Verification items for the finished model (mm, model axes). Face numbers are marked on the shaded views. A direction names the side the tool comes from. Coordinates: 2 decimals unless noted, no trailing zeros. Order: outer loops, then holes, each group sorted by start corner. A loop starts at its lowest first (then second) coordinate and runs counter-clockwise, first axis right, second up. Notation, with made-up numbers: (47, 40.25) -> (68, 40.25) arc R7 ccw to (68, 46.25) -> close; hole circle Ø11 at (81.5, 80). An arc over 180 degrees is marked (long way). Write each question's results on one line, items separated by ' | '. Start each with the question number.
(1) Cross-section at A-A on x = -0.5. Enter the section's corners in (y, z).
(2) Set-up check for the marked faces 1, 2 and 3: record each of +Z, -Z, +X, -X, +Y, -Y from which the full face is reachable in a straight line by a thin tool's end or side.
(3) Go/stop test with flat-tipped pins: pin 1 (6 mm diameter, centred on x = 32.5, y = 20, fed in from +Z); pin 2 (0.8 mm diameter, centred on y = 5.5, z = 40.5, fed in from +X); pin 3 (3 mm diameter, centred on y = 33.5, z = -12.5, fed in from -X). Record where each tip stops, or that it passes through.
(4) Cross-section at D-D on x = -16. Enter the section's corners in (y, z).
(5) Cross-section at C-C on y = 31. Enter the section's corners in (x, z), and give its area (3 significant figures).
(6) Thickness scan on probe 1 along X at (y, z) = (30.5, -0.5); probe 2 along Y at (x, z) = (18, 3.5). Record the ranges inside material, lowest first. Write a range as [from, to].
(7) Cross-section at B-B on z = 2. Enter the section's corners in (x, y).
(8) Draft check along X on the marked faces 4, 5 and 6. Enter one of: +X half, -X half, draft (parallel to the pull), parting line (faces both ways), or undercut.
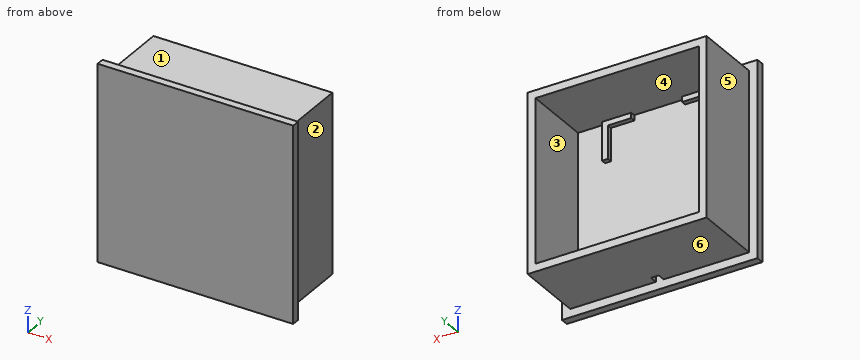
```python
from build123d import *

# Parameters (mm, degrees)
SKETCH1_W           = 100
SKETCH1_H           = 100
BOSS_EXTRUDE1_DEPTH = 4
SKETCH2_W           = 91.5
SKETCH2_H           = 91.5
SKETCH2_W_2         = 83.5
SKETCH2_H_2         = 83.5
BOSS_EXTRUDE2_DEPTH = 35
SKETCH3_W           = 4
SKETCH3_H           = 4
CUT_EXTRUDE1_DEPTH  = 4
BOSS_EXTRUDE3_DEPTH = 2.5


with BuildPart() as part:
    # Sketch1 → Boss-Extrude1 (new body)
    with BuildSketch(Plane(origin=(0, 0, 0), x_dir=(1, 0, 0), z_dir=(0, 1, 0))):
        Rectangle(SKETCH1_W, SKETCH1_H)
    extrude(amount=BOSS_EXTRUDE1_DEPTH)

    # Sketch2 → Boss-Extrude2 (add)
    with BuildSketch(Plane(origin=(0, 4, 0), x_dir=(1, 0, 0), z_dir=(0, 1, 0))):
        Rectangle(SKETCH2_W, SKETCH2_H)
        Rectangle(SKETCH2_W_2, SKETCH2_H_2, mode=Mode.SUBTRACT)
    extrude(amount=BOSS_EXTRUDE2_DEPTH)

    # Sketch3 → Cut-Extrude1 (cut)
    with BuildSketch(Plane(origin=(0, 0, -45.75), x_dir=(-1, 0, 0), z_dir=(0, 0, -1))):
        with Locations((0, 6)):
            Rectangle(SKETCH3_W, SKETCH3_H)
    extrude(amount=-CUT_EXTRUDE1_DEPTH, mode=Mode.SUBTRACT)

    # Sketch4 → Boss-Extrude3 (add)
    with BuildSketch(Plane(origin=(0, 4, 0), x_dir=(1, 0, 0), z_dir=(0, 1, 0))):
        Polygon((-28, 22.21), (-25, 22.21), (-25, 39), (-13, 39), (-13, 41.75), (-28, 41.75), align=None)
        Polygon((25, 39), (25, 22.21), (28, 22.21), (28, 41.75), (13, 41.75), (13, 39), align=None)
        Polygon((25, -39), (13, -39), (13, -41.75), (28, -41.75), (28, -22.21), (25, -22.21), align=None)
        Polygon((-13, -39), (-25, -39), (-25, -22.21), (-28, -22.21), (-28, -41.75), (-13, -41.75), align=None)
    extrude(amount=BOSS_EXTRUDE3_DEPTH)


solid = part.part
```
Results are:
1) outline: (0, -50) -> (4, -50) -> (4, 41.75) -> (39, 41.75) -> (39, 45.75) -> (4, 45.75) -> (4, 50) -> (0, 50) -> close; (8, -45.75) -> (39, -45.75) -> (39, -41.75) -> (8, -41.75) -> close
2) face 1: +Z, +X, -X, +Y | face 2: +Z, -Z, +X, +Y | face 3: +Y
3) pin 1: stops at z = 45.75 | pin 2: stops at x = 45.75 | pin 3: stops at x = -45.75
4) outline: (0, -50) -> (4, -50) -> (4, -45.75) -> (39, -45.75) -> (39, -41.75) -> (6.5, -41.75) -> (6.5, -39) -> (4, -39) -> (4, 39) -> (6.5, 39) -> (6.5, 41.75) -> (39, 41.75) -> (39, 45.75) -> (4, 45.75) -> (4, 50) -> (0, 50) -> close
5) outline: (-45.75, -45.75) -> (45.75, -45.75) -> (45.75, 45.75) -> (-45.75, 45.75) -> close; hole (-41.75, -41.75) -> (41.75, -41.75) -> (41.75, 41.75) -> (-41.75, 41.75) -> close | area: 1,400 mm2
6) probe 1: x = [-45.75, -41.75], [41.75, 45.75] | probe 2: y = [0, 4]
7) outline: (-50, 0) -> (50, 0) -> (50, 4) -> (45.75, 4) -> (45.75, 39) -> (41.75, 39) -> (41.75, 4) -> (-41.75, 4) -> (-41.75, 39) -> (-45.75, 39) -> (-45.75, 4) -> (-50, 4) -> close
8) face 4: undercut | face 5: -X half | face 6: draft
